Work out the finished part from the listing and answer in its coordinate system (mm). A direction names the side the tool comes from. Coordinates: 2 decimals unless noted, no trailing zeros. Write each question's results on one line, items separated by ' | '. Start each with the question number.
1. Which of the six approach directions +Z, -Z, +X, -X, +Y, -Y give full straight-line access (tool end or side, diameter ignored) to faces 1 (the flat face through (-0.66, 19.55, 48.84)), 2 (the cylindrical face through (0.2, 123.16, -1.51))?
2. Find the intervals of material crossed by line 1 along X through (y, z) = (174.5, 0) (3 decimals); line 2 along Z through (x, y) = (-0.25, 127); line 3 along X through (y, z) = (131, 0) (3 decimals), in increasing order. Write a range as [from, to].
3. Each of these flat-tipped pins is pushed along its axis until it touches: P1, Ø2.5, axis at x = 0, z = 0, coming from the -Y side; P2, Ø2, axis at x = 0.5, z = -1, coming from the +Y side. Where does it stop, or does it pass through?
4. Determine the mould class of faces 3 (the cylindrical face through (-3.03, 21.87, 44.51)), 4 (the cylindrical face through (-1.964, 174.581, -0.258)), 5 (the cylindrical face through (0.76, 20.62, 45.79)) for opening direction Y: released by +Y, released by -Y, zero draft, split by the parting line, or undercut.
Autodesk Inventor part; units mm, degrees
ref_plane "YZ Plane" through (0, 0, 0) normal (1, 0, 0) x (0, 1, 0)
ref_plane "XZ Plane" through (0, 0, 0) normal (0, 1, 0) x (-1, 0, 0)
sketch "Sketch1" plane through (0, 0, 0) normal (0, 1, 0) x (-1, 0, 0)
  circle A0 centre (0, 0) radius 3.175
  circle A1 centre (0, 0) radius 1.524
  dimension "d0" = 6.35
  dimension "d1" = 3.048
extrude "Extrusion1" add sketch "Sketch1" along normal blind 177.8
sketch "Sketch2" plane through (0, 177.8, 0) normal (0, 1, 0) x (1, 0, 0)
  point P0 (0, 0)
sketch "Sketch3" plane through (0, 177.8, 0) normal (0, 1, 0) x (1, 0, 0)
  point P0 (0, 0)
ref_plane "Work Plane1" through (0, 0, 3.175) normal (0, 0, 1) x (1, 0, 0)
sketch "Sketch4" plane through (0, 0, 3.175) normal (0, 0, 1) x (1, 0, 0)
  line L0 (-15.875, 25.4) -> (22.225, 25.4)
  line L1 (-15.8266, 76.2) -> (22.2734, 76.2)
  point P0 (0, 0)
  dimension "d4" = 38.1
  dimension "d5" = 25.4
  dimension "d6" = 38.1
  dimension "d7" = 76.2
bend part "Bend Part1" radius 50.8 angle 75 line through (-15.8266, 76.2, 3.175) along (1, 0, 0) centre toward (0, 0, 1) moving side (0, -1, 0) both sides no
hole "Hole1" at (0, 177.8, 0) direction (0, -1, 0) diameter 3.9624 depth 6.35
sketch "Sketch8" plane through (0, 21.5528, 49.3776) normal (0, -0.258819, 0.9659258) x (1, 0, 0)
  circle A0 centre (0, 0) radius 3.175
  circle A1 centre (0, 0) radius 1.524
  point P0 (0, -33.5983)
hole "Hole4" at (0, 21.5528, 49.3776) direction (0, 0.258819, -0.9659258) diameter 3.9624 depth 6.35
properties part number "Stainless steel tube"
Values:
1) face 1: +Z, +X, -X, -Y | face 2: +Y
2) line 1: [-3.175, -1.981], [1.981, 3.175] | line 2: [-3.17, -1.5], [1.5, 3.17] | line 3: [-3.175, -1.524], [1.524, 3.175]
3) P1: y = 54.15 | P2: y = 177.8
4) face 3: split by the parting line | face 4: zero draft | face 5: undercut
